Design review of the part shown in the three views and the two pictorial views. Dimensions are in mm from the part's minimum x, y and z. A direction names the side the tool comes from. Round coordinates to 2 decimals unless told otherwise and drop trailing zeros. Loops run counter-clockwise (first coordinate to the right, second up) from the corner with the lowest first, then second, coordinate; pieces in that order, holes last. Notation, with made-up numbers: (19.25, -27) -> (31.25, -27) arc R18 ccw to (31.25, 3) -> close; hole circle Ø8 at (-40, 36.25). An arc over 180 degrees is marked (long way). Use a Markdown table: item, result. Add a question column.
1) Wall thickness on probe 1 along X at (y, z) = (17.75, 9); probe 2 along Z at (x, y) = (30, 28.9); probe 3 along Y at (x, z) = (50.5, 19.5): over which ranges is each line inside the solid? List them lowest first.
2) Consider section A-A on x = 10.5. Give the boundary of the cut face in (y, z), plus the area to 3 significant figures.
3) Consider section C-C on z = 30. Give the boundary of the cut face in (x, y), plus the area to 3 significant figures.
4) Consider section D-D on z = 40.5. Give the boundary of the cut face in (x, y), plus the area to 3 significant figures.
5) For the marked faces 1 and 2, list the 3-axis set-ups (+Z, -Z, +X, -X, +Y, -Y) from which the entire face can be reached by the end or side of a thin tool; tool diameter is ignored.
6) Consider section B-B on y = 5. Give the boundary of the cut face in (x, z), plus the area to 3 significant figures.
7) Insertion check: pin 1 (6 mm diameter, centred on x = 25.5, z = 16, fed in from -Y). The pin has a flat end and moves straight along its axis. Give the tip position at first contact, or say it passes through.
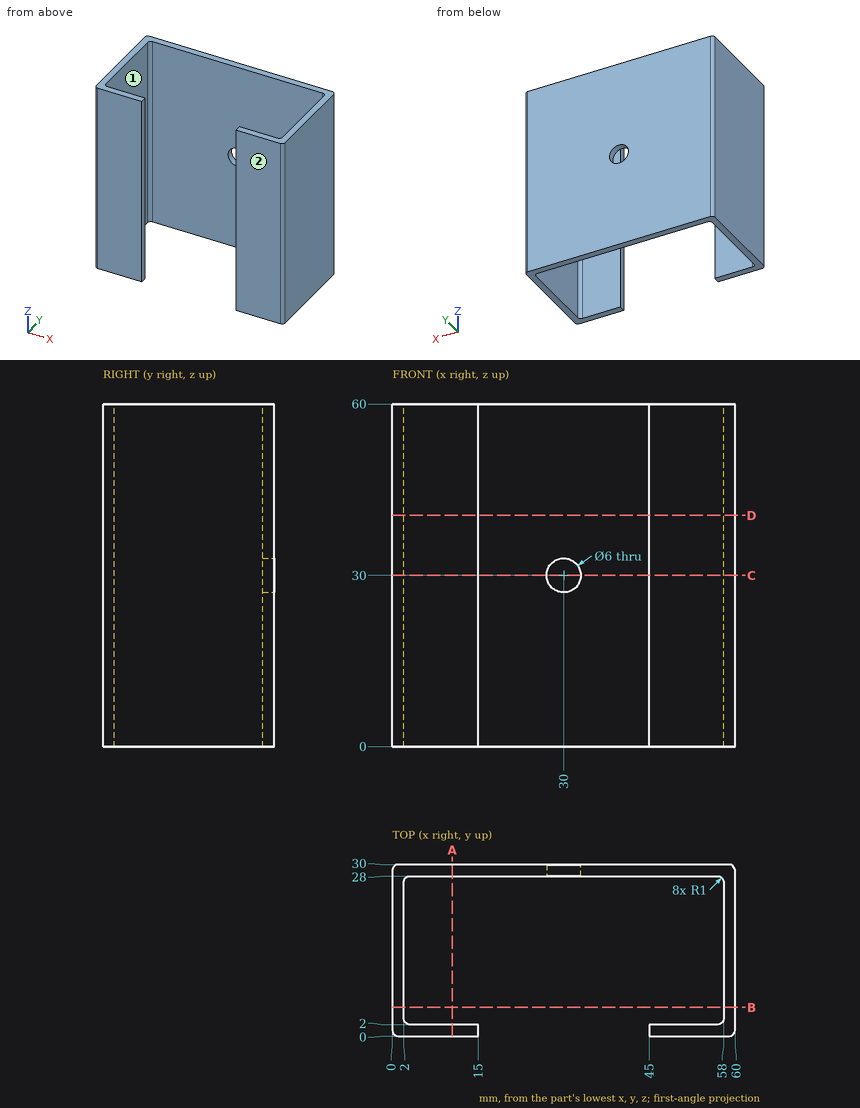
Result set:
| question | item | result |
|---|---|---|
| 1 | probe 1 | 0 to 2, 58 to 60 |
| 1 | probe 2 | 0 to 27, 33 to 60 |
| 1 | probe 3 | 0 to 2, 28 to 30 |
| 2 | outline | (0, 0) -> (2, 0) -> (2, 60) -> (0, 60) -> close; (28, 0) -> (30, 0) -> (30, 60) -> (28, 60) -> close |
| 2 | area | 240 mm2 |
| 3 | outline | (0, 1) arc R1 ccw to (1, 0) -> (15, 0) -> (15, 2) -> (3, 2) arc R1 cw to (2, 3) -> (2, 27) arc R1 cw to (3, 28) -> (27, 28) -> (27, 30) -> (1, 30) arc R1 ccw to (0, 29) -> close; (33, 28) -> (57, 28) arc R1 cw to (58, 27) -> (58, 3) arc R1 cw to (57, 2) -> (45, 2) -> (45, 0) -> (59, 0) arc R1 ccw to (60, 1) -> (60, 29) arc R1 ccw to (59, 30) -> (33, 30) -> close |
| 3 | area | 272 mm2 |
| 4 | outline | (0, 1) arc R1 ccw to (1, 0) -> (15, 0) -> (15, 2) -> (3, 2) arc R1 cw to (2, 3) -> (2, 27) arc R1 cw to (3, 28) -> (57, 28) arc R1 cw to (58, 27) -> (58, 3) arc R1 cw to (57, 2) -> (45, 2) -> (45, 0) -> (59, 0) arc R1 ccw to (60, 1) -> (60, 29) arc R1 ccw to (59, 30) -> (1, 30) arc R1 ccw to (0, 29) -> close |
| 4 | area | 284 mm2 |
| 5 | face 1 | +Z, -Z |
| 5 | face 2 | +Z, -Z, +X, -X, -Y |
| 6 | outline | (0, 0) -> (2, 0) -> (2, 60) -> (0, 60) -> close; (58, 0) -> (60, 0) -> (60, 60) -> (58, 60) -> close |
| 6 | area | 240 mm2 |
| 7 | pin 1 | y = 28 |
